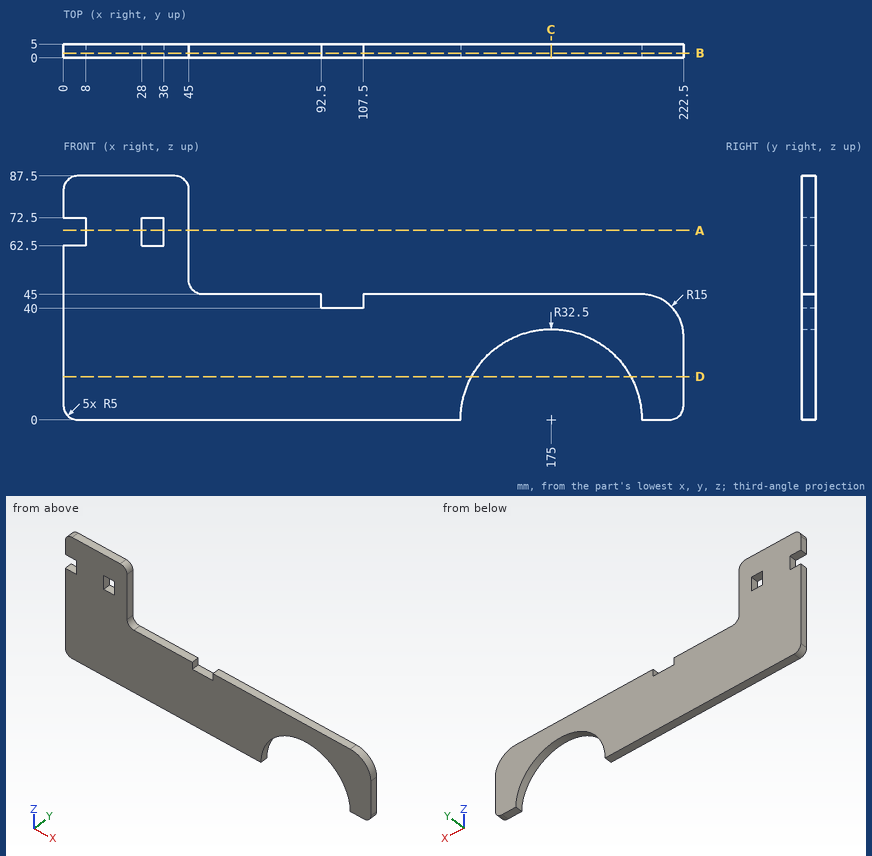
Can you work these out from the drawing? Everything is in mm from the part's minimum corner. Round coordinates to 2 decimals unless told otherwise and drop trailing zeros. Loops run counter-clockwise (first coordinate to the right, second up) from the corner with the lowest first, then second, coordinate; pieces in that order, holes last. Notation, with made-up numbers: M 37.25,-17.5 L 49.25,-17.5 A26 cw 49.25,7.5 Z; hole C 45.25,8 d8. An arc over 180 degrees is marked long. Answer in a Markdown table with one row per item.
1. Please list where these lines run through material, in increasing order: line 1 (X direction, y = 1.95, z = 67); line 2 (Z direction, x = 33.5, y = 3.7); line 3 (Z direction, x = 97, y = 2.6). Write a range as from..to.
Established:
| item | result |
|---|---|
| line 1 | 8..28, 36..45 |
| line 2 | 0..62.5, 72.5..87.5 |
| line 3 | 0..40 |
2. If we section it at B-B, the plane y = 1.7: Please give me the cut outline in (x, z), plus the area to 3 significant figures.
Established:
| item | result |
|---|---|
| outline | M 0,5 A5 ccw 5,0 L 142.5,0 A32.5 cw 207.5,0 L 217.5,0 A5 ccw 222.5,5 L 222.5,30 A15 ccw 207.5,45 L 107.5,45 L 107.5,40 L 92.5,40 L 92.5,45 L 50,45 A5 cw 45,50 L 45,82.5 A5 ccw 40,87.5 L 5,87.5 A5 ccw 0,82.5 L 0,72.5 L 8,72.5 L 8,62.5 L 0,62.5 Z; hole M 28,62.5 L 36,62.5 L 36,72.5 L 28,72.5 Z |
| area | 9,970 mm² |
3. If we section it at A-A, the plane z = 68: Please give me the cut outline in (x, y), plus the area to 3 significant figures.
Established:
| item | result |
|---|---|
| outline | M 8,0 L 28,0 L 28,5 L 8,5 Z; M 36,0 L 45,0 L 45,5 L 36,5 Z |
| area | 145 mm² |
4. If we section it at D-D, the plane z = 15.5: Please give me the cut outline in (x, y), plus the area to 3 significant figures.
Established:
| item | result |
|---|---|
| outline | M 0,0 L 146.43,0 L 146.43,5 L 0,5 Z; M 203.57,0 L 222.5,0 L 222.5,5 L 203.57,5 Z |
| area | 827 mm² |
5. If we section it at C-C, the plane x = 175: Please give me the cut outline in (y, z), plus the area to 3 significant figures.
Established:
| item | result |
|---|---|
| outline | M 0,32.5 L 5,32.5 L 5,45 L 0,45 Z |
| area | 62.5 mm² |
6. I'm going to push flat-ended pins straight in: pin 1 Ø1.5 at (x, y) = (176, 3) entering from -Z; pin 2 Ø2.5 at (y, z) = (1.5, 67.5) entering from -X; pin 3 Ø2.5 at (x, y) = (135.5, 3.5) entering from +Z. Where does each tip first touch, or does it pass through?
Established:
| item | result |
|---|---|
| pin 1 | z = 32.45 |
| pin 2 | x = 8 |
| pin 3 | z = 45 |
